Read the model definition and answer for the solid it produces. Units are mm, in the model's axes. Face numbers are marked on the shaded views. A direction names the side the tool comes from. Coordinates: 2 decimals unless noted, no trailing zeros. Loops run counter-clockwise (first coordinate to the right, second up) from the corner with the lowest first, then second, coordinate; pieces in that order, holes last. Notation, with made-up numbers: M 58,-16 L 89,-16 A12 cw 89,7 Z; hole C 79,64 d8. An arc over 180 degrees is marked long. One line per item, written item: value. Start each with the question number.
1. Consider probe 1 along Z at (x, y) = (1.45, 1.35); probe 2 along X at (y, z) = (0.8, 2.75); probe 3 along X at (y, z) = (1.9, 0). Determine where each line is inside the solid, lowest interval first.
2. Flat-ended cylindrical pins translate along their axes: pin 1 (1 mm diameter, centred on y = 0.5, z = -5, fed in from -X); pin 2 (1 mm diameter, centred on y = 0.5, z = -4, fed in from -X); pin 3 (1 mm diameter, centred on x = 0, y = 1, fed in from +Z). Find the tip coordinate at first contact, or state that the pin passes through.
3. For the marked faces 1 and 2, determine the directions among +Z, -Z, +X, -X, +Y, -Y from which every point of the face is accessible in a straight line to the end or side of a thin tool.
4. The part is cut by section C-C (z = 1.75). Write down the section's boundary in (x, y), then the cut area to 3 significant figures.
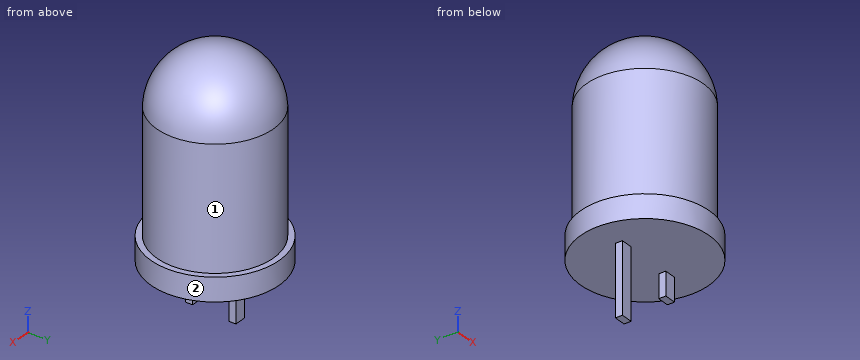
```python
from build123d import *

# Parameters (mm, degrees)
SKETCH1_R           = 2.5
BOSS_EXTRUDE1_DEPTH = 2.6
BOSS_EXTRUDE2_START = -2.6
SKETCH2_R           = 2.75
BOSS_EXTRUDE2_DEPTH = 1
DOME1_FACE_RADIUS   = 2.5
DOME1_HEIGHT        = 2.4
BOSS_EXTRUDE3_START = -3.6
SKETCH3_W           = 0.5
SKETCH3_H           = 0.3
BOSS_EXTRUDE3_DEPTH = 3
CUT_EXTRUDE1_START  = -6.6
SKETCH4_W           = 0.5
SKETCH4_H           = 0.3
CUT_EXTRUDE1_DEPTH  = 2


with BuildPart() as part:
    # Sketch1 → Boss-Extrude1 (new, symmetric)
    with BuildSketch(Plane.XY):
        Circle(SKETCH1_R)
    extrude(amount=BOSS_EXTRUDE1_DEPTH, both=True)

    # Sketch2 → Boss-Extrude2 (add)
    with BuildSketch(Plane.XY.offset(BOSS_EXTRUDE2_START)):
        Circle(SKETCH2_R)
    extrude(amount=-BOSS_EXTRUDE2_DEPTH)

    # Dome1: a dome of height H over a round flat face of radius A is a cap of a sphere of radius (A * A + H * H) / (2 * H)
    dome1_r = (DOME1_FACE_RADIUS * DOME1_FACE_RADIUS + DOME1_HEIGHT * DOME1_HEIGHT) / (2 * DOME1_HEIGHT)
    dome1_base = Plane((0, 0, 2.6), z_dir=(0, 0, 1))
    with Locations(dome1_base.offset(DOME1_HEIGHT - dome1_r)):
        dome1_ball = Sphere(dome1_r, mode=Mode.PRIVATE)
    add(split(dome1_ball, bisect_by=dome1_base, keep=Keep.TOP, mode=Mode.PRIVATE))

    # Sketch3 → Boss-Extrude3 (add)
    with BuildSketch(Plane.XY.offset(BOSS_EXTRUDE3_START)):
        with Locations((1.25, 0)):
            Rectangle(SKETCH3_W, SKETCH3_H)
        with Locations((-1.25, 0)):
            Rectangle(SKETCH3_W, SKETCH3_H)
    extrude(amount=-BOSS_EXTRUDE3_DEPTH)

    # Sketch4 → Cut-Extrude1 (cut)
    with BuildSketch(Plane.XY.offset(CUT_EXTRUDE1_START)):
        with Locations((1.25, 0)):
            Rectangle(SKETCH4_W, SKETCH4_H)
    extrude(amount=CUT_EXTRUDE1_DEPTH, mode=Mode.SUBTRACT)


solid = part.part
```
Answer block:
1. probe 1: z = -3.6 to 4.03
1. probe 2: x = -2.36 to 2.36
1. probe 3: x = -1.62 to 1.62
2. pin 1: stops at x = -1.5
2. pin 2: stops at x = -2.74
2. pin 3: stops at z = 4.95
3. face 1: +Z
3. face 2: +Z, -Z
4. outline: C 0,0 d5
4. area: 19.6 mm2
